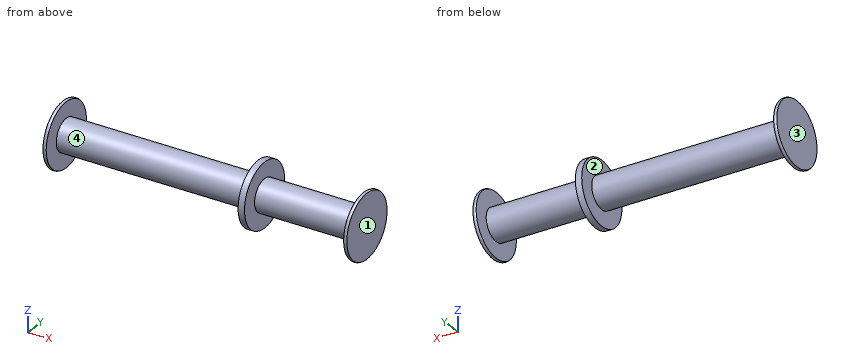
```python
from build123d import *

# Parameters (mm, degrees)
SKETCH2_R           = 10
BOSS_EXTRUDE1_DEPTH = 2


with BuildPart() as part:
    # Sketch1 → Revolve1 (revolve)
    with BuildSketch(Plane.XY):
        with BuildLine():
            Line((-47.5, 0), (47.5, 0))
            Line((47.5, 0), (47.5, -10))
            ThreePointArc((47.5, -10), (47, -10.133974596), (46.5, -10))
            Line((46.5, -10), (46.5, -5))
            Line((46.5, -5), (-46.5, -5))
            Line((-46.5, -5), (-46.5, -10))
            ThreePointArc((-46.5, -10), (-47, -10.133974596), (-47.5, -10))
            Line((-47.5, -10), (-47.5, 0))
        make_face()
    revolve(axis=Axis((-47.5, 0, 0), (1, 0, 0)))

    # Sketch2 → Boss-Extrude1 (add)
    with BuildSketch(Plane(origin=(13.5, 0, 0), x_dir=(0, 0, -1), z_dir=(1, 0, 0))):
        with Locations(Location((0, 0, 0), (0, 0, 90))):
            Circle(SKETCH2_R)
    extrude(amount=BOSS_EXTRUDE1_DEPTH)


solid = part.part
```
Geometry check sheet. Reference: the model listing, model coordinates, mm. Face numbers are marked on the shaded views. Give positions to 0.01 mm unless a question says otherwise; leave off trailing zeros. Order: outer loops, then holes, each group sorted by start corner. A loop starts at its lowest first (then second) coordinate and runs counter-clockwise, first axis right, second up.
1. Section check C-C, the plane y = 8. Give the number of separate pieces and of enclosed holes in the cut face, and give its area (3 significant figures).
2. Gauge pin test, flat ends, axial feed: pin 1 Ø1.5 at (x, y) = (16, -4.5) entering from -Z; pin 2 Ø3 at (x, y) = (14, -6.5) entering from -Z; pin 3 Ø4 at (x, z) = (-16, 5.5) entering from +Y. Record the tip position at first contact, or that the pin passes through.
3. Section check A-A, the plane z = 0. Enter the section's corners in (x, y), and give its area (3 significant figures).
4. Release check for a two-part mould opening along X. For the marked faces 1, 2, 3 and 4 record: pulls with the +X half, pulls with the -X half, needs draft (parallel to the pull), parting line crosses it, or undercut.
5. Thickness scan on L1, parallel to X at y = 7.5, z = 1; L2, parallel to Z at x = -36, y = 0.25; L3, parallel to Z at x = 2, y = 1.5. Record the ranges inside material, lowest first.
6. Section check D-D, the plane x = 1.5. Enter the section's corners in (y, z).
Values follow:
1. separate pieces: 3
1. enclosed holes: 0
1. area: 48.6 mm2
2. pin 1: stops at z = -9.19
2. pin 2: stops at z = -8.66
2. pin 3: stops at y = 3.57
3. outline: (-47.5, -10) arc R1 ccw to (-46.5, -10) - (-46.5, -5) - (13.5, -5) - (13.5, -10) - (15.5, -10) - (15.5, -5) - (46.5, -5) - (46.5, -10) arc R1 ccw to (47.5, -10) - (47.5, 10) arc R1 ccw to (46.5, 10) - (46.5, 5) - (15.5, 5) - (15.5, 10) - (13.5, 10) - (13.5, 5) - (-46.5, 5) - (-46.5, 10) arc R1 ccw to (-47.5, 10) - close
3. area: 990 mm2
4. face 1: pulls with the +X half
4. face 2: undercut
4. face 3: pulls with the -X half
4. face 4: undercut
5. L1: x = -47.5 to -46.5, 13.5 to 15.5, 46.5 to 47.5
5. L2: z = -4.99 to 4.99
5. L3: z = -4.77 to 4.77
6. outline: circle Ø10 at (0, 0)
